from build123d import *

# Parameters (mm, degrees)
CHAMFER1_SIZE      = 3
SKETCH2_W          = 6
SKETCH2_H          = 6
CUT_EXTRUDE1_DEPTH = 116


with BuildPart() as part:
    # Sketch1 → Revolve1 (revolve)
    with BuildSketch(Plane.XY):
        Polygon((57.5, 12.5), (-57.5, 12.5), (-57.5, 22.5), (-37.5, 22.5), (-37.5, 42.5), (-29.5, 42.5), (-24, 27.5), (-19, 27.5), (-13.5, 50), (-8.5, 50), (-3, 35), (2, 35), (7.5, 57.5), (12.5, 57.5), (18, 42.5), (23, 42.5), (28.5, 65), (33.5, 65), (39, 52.5), (44, 52.5), (49.5, 65), (57.5, 65), (57.5, 47.5), (12.5, 27.5), (12.5, 22.5), (57.5, 22.5), align=None)
    revolve(axis=Axis((57.5, 0, 0), (-1, 0, 0)))

    # Chamfer1
    chamfer1_edges = [part.edges().sort_by_distance(p)[0] for p in [
        (57.5, -65, 0),
        (-37.5, -42.5, 0),
    ]]
    chamfer(chamfer1_edges, length=CHAMFER1_SIZE)

    # Sketch2 → Cut-Extrude1 (cut, through all)
    with BuildSketch(Plane.ZY.offset(57.5)):
        with Locations((0, -12.5)):
            Rectangle(SKETCH2_W, SKETCH2_H)
    extrude(amount=-CUT_EXTRUDE1_DEPTH, mode=Mode.SUBTRACT)


solid = part.part
Source: CAD feature listing. Evaluate the final solid. Frame: model axes, mm. A direction names the side the tool comes from. Round coordinates to 2 decimals unless told otherwise and drop trailing zeros. Loops run counter-clockwise (first coordinate to the right, second up) from the corner with the lowest first, then second, coordinate; pieces in that order, holes last. Notation, with made-up numbers: (38, -18) -> (83, -18) arc R33 cw to (83, 21) -> close; hole circle Ø5 at (51.25, 44). An arc over 180 degrees is marked (long way). Answer as a JSON object with one key per item and string values. Group by question number.
Q1. Section query A-A (x = 30.5). Output: boundary loops of the cut face in (y, z).
Q2. Section query B-B (x = 47). Output: boundary loops of the cut face in (y, z).
Q3. Ray query, line 1 (X direction, y = -17, z = 45); line 2 (X direction, y = 19, z = -42); line 3 (Y direction, x = -2.5, z = -1). Return the intervals inside material, ascending. Write a range as from..to.
Q4. Access query for faces 5 (the flat face through (57.5, 10, 10)), 6 (the cylindrical face through (-47.36, 10.382, 19.961)), 7 (the cylindrical face through (35.315, 10.382, 19.961)), 8 (the conical face through (23.344, 23.604, -37.023)), 9 (the flat face through (-1, -14, 3)). Directions: +Z, -Z, +X, -X, +Y, -Y. A direction counts if a zero-diameter tool reaches every point of the face in a straight line with its end or side. Return the directions, or none.
Q5. Mould query, pull axis Y, two halves, no side actions, for faces 1 (the flat face through (-1, -14, -3)), 2 (the flat face through (-57.5, -10, 10)), 3 (the cylindrical face through (20.535, -33.727, 25.861)), 4 (the flat face through (-1, -15.5, 0)). Classes: pulls with the +Y half, pulls with the -Y half, needs draft (parallel to the pull), parting line crosses it, or undercut.
Q6. Section query C-C (y = -55.5). State how many separate pieces and enclosed holes the cut face has, plus the area to 3 significant figures.
Q7. Contact query for flat-ended pins moving along their axis: P1, Ø2, axis at x = -13.5, y = -12.5, coming from the +Z side; P2, Ø10, axis at x = 30.5, y = -6, coming from the -Z side; P3, Ø3, axis at x = 32, y = -39.5, coming from the +Z side. Output: stop coordinate, or through.
Completed:
{
 "1": {"outline": "circle Ø130 at (0, 0); circle Ø45 at (0, 0); hole circle Ø71 at (0, 0); hole (-15.5, -3) -> (-12.13, -3) arc R12.5 ccw (long way) to (-12.13, 3) -> (-15.5, 3) -> close"},
 "2": {"outline": "circle Ø118.64 at (0, 0); circle Ø45 at (0, 0); hole circle Ø85.67 at (0, 0); hole (-15.5, -3) -> (-12.13, -3) arc R12.5 ccw (long way) to (-12.13, 3) -> (-15.5, 3) -> close"},
 "3": {"line 1": "-13.96..-7.8, 5.2..15.95, 24.37..57.5", "line 2": "-14.45..-7.07, 4.71..16.68, 23.88..54.34", "line 3": "-34.99..-15.5, 12.46..34.99"},
 "4": {"face 5": "+Z, -Z, +X, +Y, -Y", "face 6": "-X", "face 7": "+X", "face 8": "none", "face 9": "+X, -X"},
 "5": {"face 1": "undercut", "face 2": "needs draft", "face 3": "parting line crosses it", "face 4": "undercut"},
 "6": {"separate pieces": "3", "enclosed holes": "0", "area": "1,510 mm²"},
 "7": {"P1": "z = 48.66", "P2": "z = -64.99", "P3": "z = 52.74"}
}
